Geometry check sheet. Reference: the model listing, model coordinates, mm. A direction names the side the tool comes from. Round coordinates to 2 decimals unless told otherwise and drop trailing zeros. Order: outer loops, then holes, each group sorted by start corner. A loop starts at its lowest first (then second) coordinate and runs counter-clockwise, first axis right, second up.
```python
from build123d import *

# Parameters (mm, degrees)
F2_R      = 2.5
F3_DEPTH  = 3
F4_W      = 3
F4_H      = 35
F4_H_2    = 3
F4_W_2    = 41
F5_DEPTH  = 114
F6_R      = 2.5
F7_DEPTH  = 3
F8_W      = 110
F8_H      = 20
F9_DEPTH  = 3
F10_W     = 47
F10_H     = 26
F10_W_2   = 48
F10_H_2   = 28
F11_DEPTH = 3
F12_SIZE  = 1
F14_W     = 48
F14_H     = 2
F14_W_2   = 47
F15_DEPTH = 1
F16_DEPTH = 26


with BuildPart() as f3:
    # F2 (on Right) → F3 (new body)
    with BuildSketch(Plane.YZ):
        with BuildLine():
            ThreePointArc((22.5, 35), (21.0355339059, 38.5355339059), (17.5, 40))
            Line((17.5, 40), (-19.5, 40))
            ThreePointArc((-19.5, 40), (-23.0355339059, 38.5355339059), (-24.5, 35))
            Line((-24.5, 35), (-24.5, -38))
            Line((-24.5, -38), (22.5, -38))
            Line((22.5, -38), (22.5, 35))
        make_face()
        with Locations((-12, 34.5)):
            Circle(F2_R, mode=Mode.SUBTRACT)
        with Locations((10, 34.5)):
            Circle(F2_R, mode=Mode.SUBTRACT)
    extrude(amount=F3_DEPTH)

    # F4 (on Right) → F5 (join)
    with BuildSketch(Plane.YZ):
        with Locations((-23, -17.5)):
            Rectangle(F4_W, F4_H)
        with Locations((21, -36.5)):
            Rectangle(F4_W, F4_H_2)
        with Locations((21, -17.5)):
            Rectangle(F4_W, F4_H)
        with Locations((-1, -36.5)):
            Rectangle(F4_W_2, F4_H_2)
        with Locations((-23, -36.5)):
            Rectangle(F4_W, F4_H_2)
    extrude(amount=-F5_DEPTH)

    # F6 (on face) → F7 (join)
    with BuildSketch(Plane(origin=(-114, 0, 0), x_dir=(0, -1, 0), z_dir=(-1, 0, 0))):
        with BuildLine():
            ThreePointArc((24.5, 35), (23.0355339059, 38.5355339059), (19.5, 40))
            Line((19.5, 40), (-17.5, 40))
            ThreePointArc((-17.5, 40), (-21.0355339059, 38.5355339059), (-22.5, 35))
            Line((-22.5, 35), (-22.5, -38))
            Line((-22.5, -38), (24.5, -38))
            Line((24.5, -38), (24.5, 35))
        make_face()
        with Locations((-10, 34.5)):
            Circle(F6_R, mode=Mode.SUBTRACT)
    extrude(amount=F7_DEPTH)

    # F8 (on face) → F9 (join)
    with BuildSketch(Plane.XZ.offset(24.5)):
        with Locations((-57, 10)):
            Rectangle(F8_W, F8_H)
    extrude(amount=-F9_DEPTH)

    # F10 (on face) → F11 (cut, through all)
    with BuildSketch(Plane.XZ.offset(24.5)):
        with Locations((-85.5, -19)):
            Rectangle(F10_W, F10_H)
        with Locations((-28.5, -19)):
            Rectangle(F10_W_2, F10_H_2)
    extrude(amount=-F11_DEPTH, mode=Mode.SUBTRACT)

    # F12
    f12_edges = [f3.edges().sort_by_distance(p)[0] for p in [
        (-57, -24.5, -38),
        (3, -1, -38),
        (-57, 22.5, -38),
        (-117, -1, -38),
    ]]
    chamfer(f12_edges, length=F12_SIZE)

    # F14 (on face) → F15 (cut)
    with BuildSketch(Plane(origin=(0, -21.5, 0), x_dir=(-1, 0, 0), z_dir=(0, 1, 0))):
        with Locations((28.5, -34)):
            Rectangle(F14_W, F14_H)
        with Locations((85.5, -33)):
            Rectangle(F14_W_2, F14_H)
        with Locations((85.5, -5)):
            Rectangle(F14_W_2, F14_H)
        with Locations((28.5, -4)):
            Rectangle(F14_W, F14_H)
    extrude(amount=-F15_DEPTH, mode=Mode.SUBTRACT)

    # F16 (add): a face of the model
    f16_faces = [f3.faces().sort_by_distance(p)[0] for p in [
        (-85.5, -23.5, -32),
    ]]
    extrude(f16_faces, amount=F16_DEPTH)


solid = f3.part
```
(1) Set-up check for faces 4 (the flat face through (-85, -22.5, -19)), 5 (the cylindrical face through (1, -14, 36)), 6 (the flat face through (-56, -21.5, 4)), 7 (the flat face through (-58, -23, 20)): record each of +Z, -Z, +X, -X, +Y, -Y from which the full face is reachable in a straight line by a thin tool's end or side.
Returned:
face 4: none
face 5: +X
face 6: +Z
face 7: +Z, +Y, -Y
(2) Sectioned sample at A-A, the plane y = 10. Record the cut outline in (x, z), and give its area (3 significant figures).
Returned:
outline: (-117, -37) - (-116, -38) - (2, -38) - (3, -37) - (3, 32) - (0, 32) - (0, -35) - (-114, -35) - (-114, 32) - (-117, 32) - close; (-117, 37) - (-114, 37) - (-114, 40) - (-117, 40) - close; (0, 37) - (3, 37) - (3, 40) - (0, 40) - close
area: 779 mm2
(3) Material ranges on line 1 (X direction, y = 12, z = -16.5); line 2 (Z direction, x = -115.35, y = 10); line 3 (Z direction, x = -85.5, y = -8.5), recorded low to high.
Returned:
line 1: x = -117 to -114, 0 to 3
line 2: z = -38 to 32, 37 to 40
line 3: z = -38 to -35
(4) Sectioned sample at C-C, the plane z = 8.5. Record the cut outline in (x, y), and give its area (3 significant figures).
Returned:
outline: (-117, -24.5) - (-114, -24.5) - (-114, 22.5) - (-117, 22.5) - close; (-112, -24.5) - (-2, -24.5) - (-2, -21.5) - (-112, -21.5) - close; (0, -24.5) - (3, -24.5) - (3, 22.5) - (0, 22.5) - close
area: 612 mm2
(5) Draft check along Z on faces 1 (the cylindrical face through (1.48, 11.34, 36.61)), 2 (the flat face through (-56, -1, -38)), 3 (the flat face through (-71, -24.5, -10)). Enter one of: released by +Z, released by -Z, zero draft, split by the parting line, or undercut.
Returned:
face 1: undercut
face 2: released by -Z
face 3: zero draft
(6) Sectioned sample at D-D, the plane y = -12. Record the cut outline in (x, z), and give its area (3 significant figures).
Returned:
outline: (-117, -37) - (-116, -38) - (2, -38) - (3, -37) - (3, 32) - (0, 32) - (0, -35) - (-114, -35) - (-114, 40) - (-117, 40) - close; (0, 37) - (3, 37) - (3, 40) - (0, 40) - close
area: 794 mm2
(7) Sectioned sample at B-B, the plane x = -41. Record the cut outline in (y, z), and give its area (3 significant figures).
Returned:
outline: (-24.5, -37) - (-23.5, -38) - (21.5, -38) - (22.5, -37) - (22.5, 0) - (19.5, 0) - (19.5, -35) - (-22.5, -35) - (-22.5, -33) - (-24.5, -33) - close; (-24.5, -5) - (-22.5, -5) - (-22.5, -3) - (-21.5, -3) - (-21.5, 20) - (-24.5, 20) - close
area: 322 mm2
(8) Depth check by flat-ended pin: P1, Ø1.6, axis at x = -30.5, y = -24, coming from the +Z side; P2, Ø6, axis at x = -49.5, z = 20, coming from the +Y side; P3, Ø4, axis at y = -12, z = 34.5, coming from the +X side. Enter the tip coordinate at first touch or a pass-through.
Returned:
P1: stops at z = 20
P2: stops at y = -21.5
P3: stops at x = -114
